from build123d import *

# Parameters (mm, degrees)
SKETCH1_W           = 87.5
SKETCH1_H           = 42
BOSS_EXTRUDE1_DEPTH = 5
SKETCH2_W           = 87.5
SKETCH2_H           = 1
CUT_EXTRUDE1_DEPTH  = 3
SKETCH3_W           = 87.5
SKETCH3_H           = 1
CUT_EXTRUDE2_DEPTH  = 3
SKETCH4_W           = 10
SKETCH4_H           = 20
CUT_EXTRUDE3_DEPTH  = 1
FILLET1_R           = 10
FILLET2_R           = 10
SHELL6_START        = -41.25
SHELL6_DEPTH        = 82.5
SHELL6_2_DEPTH      = 33.75
SHELL6_START_2      = 7.5
SHELL6_3_DEPTH      = 33.75
SKETCH5_R           = 3
CUT_EXTRUDE4_DEPTH  = 2.5
LPATTERN1_COUNT     = 3
LPATTERN1_PITCH     = 11


# Read off the part's stored shape, not the designer's step: Shell6
with BuildPart() as part:
    # Sketch1 → Boss-Extrude1 (new body)
    with BuildSketch(Plane(origin=(0, 0, 0), x_dir=(1, 0, 0), z_dir=(0, 1, 0))):
        Rectangle(SKETCH1_W, SKETCH1_H)
    extrude(amount=BOSS_EXTRUDE1_DEPTH)

    # Sketch2 → Cut-Extrude1 (cut)
    with BuildSketch(Plane(origin=(0, 5, 0), x_dir=(1, 0, 0), z_dir=(0, 1, 0))):
        with Locations((0, 20.5)):
            Rectangle(SKETCH2_W, SKETCH2_H)
    extrude(amount=-CUT_EXTRUDE1_DEPTH, mode=Mode.SUBTRACT)

    # Sketch3 → Cut-Extrude2 (cut)
    with BuildSketch(Plane(origin=(0, 5, 0), x_dir=(1, 0, 0), z_dir=(0, 1, 0))):
        with Locations((0, -20.5)):
            Rectangle(SKETCH3_W, SKETCH3_H)
    extrude(amount=-CUT_EXTRUDE2_DEPTH, mode=Mode.SUBTRACT)

    # Sketch4 → Cut-Extrude3 (cut)
    with BuildSketch(Plane(origin=(0, 5, 0), x_dir=(1, 0, 0), z_dir=(0, 1, 0))):
        Rectangle(SKETCH4_W, SKETCH4_H)
    extrude(amount=-CUT_EXTRUDE3_DEPTH, mode=Mode.SUBTRACT)

    # Fillet1
    # the kernel refuses this fillet: 10 mm, written as the material it adds along each edge
    with BuildSketch(Plane(origin=(15.897247359, 4, 10), x_dir=(0, 1, 0), z_dir=(-1, 0, 0))) as fillet1_piece_1:
        with BuildLine():
            CenterArc((10, 4.358898944), FILLET1_R, 180, 25.841932763)
            Line((0, 4.358898944), (-0.2, 4.358898944))
            Line((-0.2, 4.358898944), (-0.2, 0))
            Line((-0.2, 0), (0, -0.2))
            ThreePointArc((0, -0.2), (0.5, -0.2), (0.82, -0.087177979))
            Line((0.82, -0.087177979), (1, 0))
        make_face()
    extrude(amount=31.794494718)

    # Fillet2
    # the kernel refuses this fillet: 10 mm, written as the material it adds along each edge
    with BuildSketch(Plane(origin=(-15.897247359, 4, -10), x_dir=(0, 0, 1), z_dir=(1, 0, 0))) as fillet2_piece_1:
        with BuildLine():
            CenterArc((4.358898944, -10), FILLET2_R, 90, 25.841932763)
            Line((0, -1), (-0.087177979, -0.82))
            ThreePointArc((-0.087177979, -0.82), (-0.2, -0.5), (-0.2, 0))
            Line((-0.2, 0), (0, 0.2))
            Line((0, 0.2), (4.358898944, 0.2))
            Line((4.358898944, 0.2), (4.358898944, 0))
        make_face()
    extrude(amount=31.794494718)

    # Shell6 outline → Shell6 (cut)
    with BuildSketch(Plane.YZ.offset(SHELL6_START)):
        with BuildLine():
            Line((0, -17.5), (2.5, -17.5))
            Line((2.5, -17.5), (2.5, -10.540080542))
            ThreePointArc((2.5, -10.540080542), (1.752551286, -8.141101056), (1.5, -5.641101056))
            Line((1.5, -5.641101056), (1.5, 5.641101056))
            ThreePointArc((1.5, 5.641101056), (1.752551286, 8.141101056), (2.5, 10.540080542))
            Line((2.5, 10.540080542), (2.5, 17.5))
            Line((2.5, 17.5), (0, 17.5))
            Line((0, 17.5), (0, -17.5))
        make_face()
    extrude(amount=SHELL6_DEPTH, mode=Mode.SUBTRACT)

    # Shell6 2 outline → Shell6 2 (cut)
    with BuildSketch(Plane.YZ.offset(SHELL6_START)):
        with BuildLine():
            ThreePointArc((1.5, -5.641101056), (1.752551286, -8.141101056), (2.5, -10.540080542))
            Line((2.5, -10.540080542), (2.5, 10.540080542))
            ThreePointArc((2.5, 10.540080542), (1.752551286, 8.141101056), (1.5, 5.641101056))
            Line((1.5, 5.641101056), (1.5, -5.641101056))
        make_face()
    extrude(amount=SHELL6_2_DEPTH, mode=Mode.SUBTRACT)

    # Shell6 3 outline → Shell6 3 (cut)
    with BuildSketch(Plane.YZ.offset(SHELL6_START_2)):
        with BuildLine():
            ThreePointArc((1.5, -5.641101056), (1.752551286, -8.141101056), (2.5, -10.540080542))
            Line((2.5, -10.540080542), (2.5, 10.540080542))
            ThreePointArc((2.5, 10.540080542), (1.752551286, 8.141101056), (1.5, 5.641101056))
            Line((1.5, 5.641101056), (1.5, -5.641101056))
        make_face()
    extrude(amount=SHELL6_3_DEPTH, mode=Mode.SUBTRACT)

    # Sketch5 → Cut-Extrude4 (cut)
    with BuildSketch(Plane(origin=(0, 5, 0), x_dir=(1, 0, 0), z_dir=(0, 1, 0))):
        with Locations(Location((-35.01329609, 10, 0), (0, 0, 270))):
            Circle(SKETCH5_R)
        with Locations(Location((-35.01329609, -10, 0), (0, 0, 270))):
            Circle(SKETCH5_R)
        with Locations(Location((11.17688744, 10, 0), (0, 0, 270))):
            Circle(SKETCH5_R)
        with Locations(Location((11.17688744, -10, 0), (0, 0, 270))):
            Circle(SKETCH5_R)
    cut_extrude4 = extrude(amount=-CUT_EXTRUDE4_DEPTH, mode=Mode.SUBTRACT)

    # LPattern1: Cut-Extrude4 ×3
    with Locations(*[(i * LPATTERN1_PITCH, 0, 0) for i in range(1, LPATTERN1_COUNT)]):
        add(cut_extrude4, mode=Mode.SUBTRACT)


solid = part.part
Work out the finished part from the listing and answer in its coordinate system (mm). A direction names the side the tool comes from. Give positions to 0.01 mm unless a question says otherwise; leave off trailing zeros. Write each loop counter-clockwise with the first axis right and the second up, starting at its lowest first coordinate (ties: lowest second). Pieces come first, ordered by that corner, then holes.
Q1. A tool of negligible diameter and unlimited length cuts with its end or side. For faces 1 (the face through (-0.11, 1.76, -8.18)), 2 (the face through (30.515, 3.768, 11.384)), from which of +Z, -Z, +X, -X, +Y, -Y can it reach the whole face along a straight path? Write none if from no direction.
Answer:
face 1: -Y
face 2: +Y, -Y
Q2. The part is cut by section B-B on x = -36.5. Give the vertices of the cut face in (y, z).
Answer:
outline: (0, -21) - (2, -21) - (2, -20) - (5, -20) - (5, -12.61) - (2.5, -12.61) - (2.5, -17.5) - (0, -17.5) - close; (0, 17.5) - (2.5, 17.5) - (2.5, 12.61) - (5, 12.61) - (5, 20) - (2, 20) - (2, 21) - (0, 21) - close; (2.5, -7.39) - (5, -7.39) - (5, 7.39) - (2.5, 7.39) - close
Q3. The part is cut by section A-A on x = 24. Give the vertices of the cut face in (y, z), and give its area (3 significant figures).
Answer:
outline: (0, -21) - (2, -21) - (2, -20) - (5, -20) - (5, -12.38) - (2.5, -12.38) - (2.5, -17.5) - (0, -17.5) - close; (0, 17.5) - (2.5, 17.5) - (2.5, 12.38) - (5, 12.38) - (5, 20) - (2, 20) - (2, 21) - (0, 21) - close; (2.5, -7.62) - (5, -7.62) - (5, 7.62) - (2.5, 7.62) - close
area: 92.7 mm2
Q4. Given pin 1 (5 mm diameter, centred on x = -35.01, z = -10, fed in from +Y); pin 2 (7 mm diameter, centred on x = -24.01, z = -10, fed in from -Y); pin 3 (0.5 mm diameter, centred on x = 1.5, z = 20.5, fed in from +Y); pin 4 (0.9 mm diameter, centred on x = 9.5, y = 3, fed in from -Z), each flat-ended and moving along its own axis, determine where each tip first touches the part or whether it passes through.
Answer:
pin 1: passes through
pin 2: stops at y = 2.5
pin 3: stops at y = 2
pin 4: stops at z = -20
Q5. Straight lines are drawn through the part: L1, parallel to X at y = 2.15, z = -11; L2, parallel to Z at x = 3.5, y = 0.9; L3, parallel to Z at x = -26.5, y = 2.95. For each, find the intervals that lie inside material, in ascending order.
Answer:
L1: x = -43.75 to -41.25, 41.25 to 43.75
L2: z = -21 to -17.5, 17.5 to 21
L3: z = -20 to -11.68, -8.32 to 8.32, 11.68 to 20
Q6. For a pull along X with two mould halves and no side action, classify faces 3 (the face through (-15.94, 3.77, -10.65)), 4 (the face through (-1, 1, 17.5)), 5 (the face through (-1, 4, 20)), 6 (the face through (-43.75, 2, 0)) as released by +X, released by -X, zero draft, split by the parting line, or undercut.
Answer:
face 3: undercut
face 4: undercut
face 5: zero draft
face 6: released by -X
